Geometry check sheet. Reference: drawing and pictorial views, mm from the part's lowest x, y, z. Round coordinates to 2 decimals unless told otherwise and drop trailing zeros. Order: outer loops, then holes, each group sorted by start corner. A loop starts at its lowest first (then second) coordinate and runs counter-clockwise, first axis right, second up. Notation, with made-up numbers: M 14.5,46.5 L 43.5,46.5 A15 cw 43.5,60.5 Z; hole C 11,73.25 d5. An arc over 180 degrees is marked long. Answer as a JSON object with one key per item and string values. Group by question number.
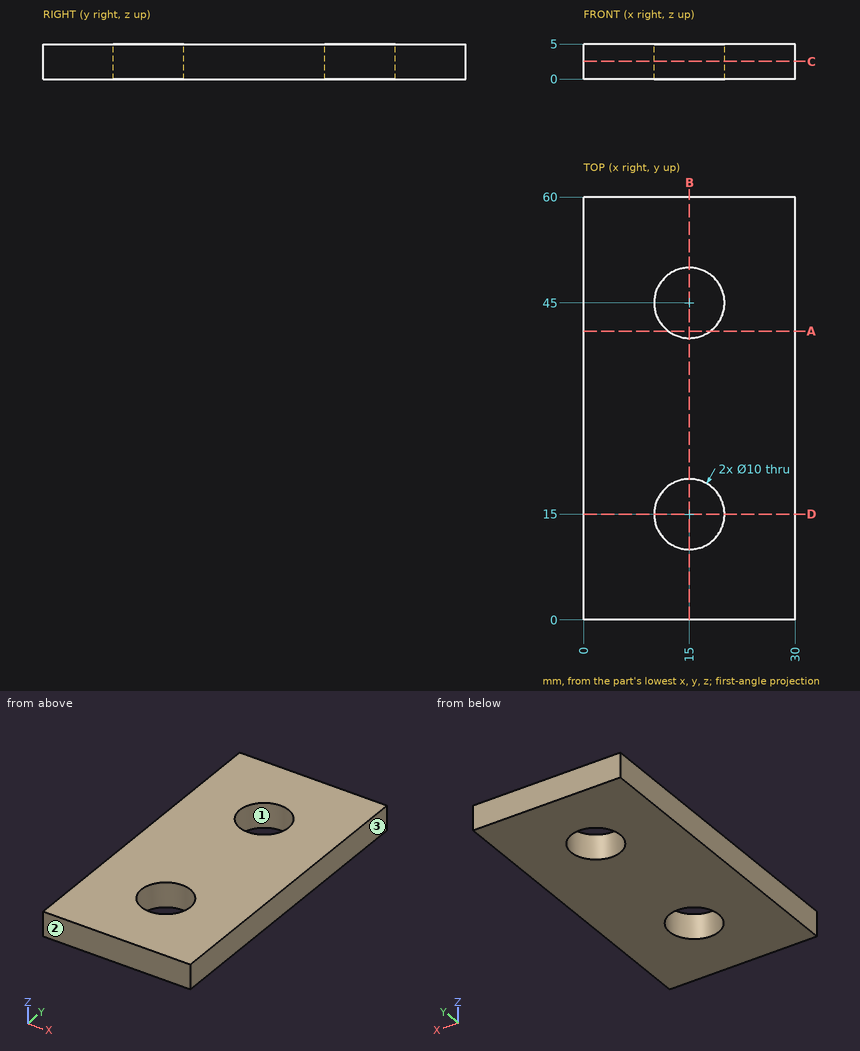
Q1. Cross-section at B-B, the plane x = 15. Record the cut outline in (y, z).
Q2. Cross-section at D-D, the plane y = 15. Record the cut outline in (x, z), then the cut area to 3 significant figures.
Q3. Thickness scan on line 1 (Y direction, x = 15, z = 2.3); line 2 (Y direction, x = 18.75, z = 1.7); line 3 (X direction, y = 18, z = 1.15). Record the ranges inside material, lowest first. Write a range as from..to.
Q4. Release check for a two-part mould opening along X. For the marked faces 1, 2 and 3 record: released by +X, released by -X, zero draft, split by the parting line, or undercut.
Q5. Gauge pin test, flat ends, axial feed: pin 1 Ø3 at (x, z) = (17, 4) entering from -Y; pin 2 Ø9 at (x, y) = (15, 45) entering from -Z. Record the tip position at first contact, or that the pin passes through.
Q6. Cross-section at A-A, the plane y = 41. Record the cut outline in (x, z), then the cut area to 3 significant figures.
Q7. Cross-section at C-C, the plane z = 2.55. Record the cut outline in (x, y), then the cut area to 3 significant figures.
Conclusion:
{
 "1": {"outline": "M 0,0 L 10,0 L 10,5 L 0,5 Z; M 20,0 L 40,0 L 40,5 L 20,5 Z; M 50,0 L 60,0 L 60,5 L 50,5 Z"},
 "2": {"outline": "M 0,0 L 10,0 L 10,5 L 0,5 Z; M 20,0 L 30,0 L 30,5 L 20,5 Z", "area": "100 mm2"},
 "3": {"line 1": "0..10, 20..40, 50..60", "line 2": "0..11.69, 18.31..41.69, 48.31..60", "line 3": "0..11, 19..30"},
 "4": {"face 1": "undercut", "face 2": "zero draft", "face 3": "released by +X"},
 "5": {"pin 1": "y = 0", "pin 2": "through"},
 "6": {"outline": "M 0,0 L 12,0 L 12,5 L 0,5 Z; M 18,0 L 30,0 L 30,5 L 18,5 Z", "area": "120 mm2"},
 "7": {"outline": "M 0,0 L 30,0 L 30,60 L 0,60 Z; hole C 15,15 d10; hole C 15,45 d10", "area": "1,640 mm2"}
}
